Check sheet for the modelled part. Datum: model origin and axes. Units: mm. Face numbers are marked on the shaded views. Give positions to 0.01 mm unless a question says otherwise; leave off trailing zeros. Order: outer loops, then holes, each group sorted by start corner. A loop starts at its lowest first (then second) coordinate and runs counter-clockwise, first axis right, second up.
```python
from build123d import *

# Parameters (mm, degrees)
SKETCH1_R           = 10.308435719
BOSS_EXTRUDE1_DEPTH = 6


with BuildPart() as part:
    # Sketch1 → Boss-Extrude1 (new body)
    with BuildSketch(Plane(origin=(0, 0, 0), x_dir=(1, 0, 0), z_dir=(0, 1, 0))):
        Polygon((9.406647228, 13.324720403), (37.205859161, 61.474367881), (61.474367881, 37.205859161), (13.324720403, 9.406647228), (14.808755665, 6.836222753), (62.958403143, 34.635434686), (71.841293847, 1.484035262), (16.242869981, 1.484035262), (16.242869981, -1.484035262), (71.841293847, -1.484035262), (62.958403143, -34.635434686), (14.808755665, -6.836222753), (13.324720403, -9.406647228), (61.474367881, -37.205859161), (37.205859161, -61.474367881), (9.406647228, -13.324720403), (6.836222753, -14.808755665), (34.635434686, -62.958403143), (1.484035262, -71.841293847), (1.484035262, -16.242869981), (-1.484035262, -16.242869981), (-1.484035262, -71.841293847), (-34.635434686, -62.958403143), (-6.836222753, -14.808755665), (-9.406647228, -13.324720403), (-37.205859161, -61.474367881), (-61.474367881, -37.205859161), (-13.324720403, -9.406647228), (-14.808755665, -6.836222753), (-62.958403143, -34.635434686), (-71.841293847, -1.484035262), (-16.242869981, -1.484035262), (-16.242869981, 1.484035262), (-71.841293847, 1.484035262), (-62.958403143, 34.635434686), (-14.808755665, 6.836222753), (-13.324720403, 9.406647228), (-61.474367881, 37.205859161), (-37.205859161, 61.474367881), (-9.406647228, 13.324720403), (-6.836222753, 14.808755665), (-34.635434686, 62.958403143), (-1.484035262, 71.841293847), (-1.484035262, 16.242869981), (1.484035262, 16.242869981), (1.484035262, 71.841293847), (34.635434686, 62.958403143), (6.836222753, 14.808755665), align=None)
        with Locations(Location((0, 0, 0), (0, 0, 270))):
            Circle(SKETCH1_R, mode=Mode.SUBTRACT)
    extrude(amount=-BOSS_EXTRUDE1_DEPTH)


solid = part.part
```
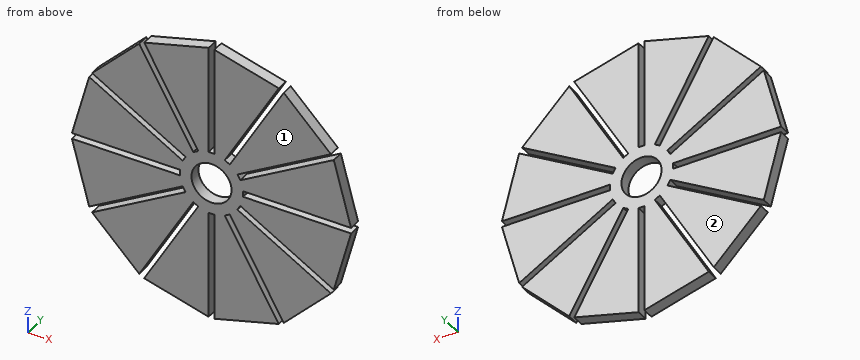
(1) Gauge pin test, flat ends, axial feed: pin 1 Ø3.5 at (y, z) = (-2, 0) entering from +X; pin 2 Ø0.9 at (x, y) = (0.5, -3) entering from -Z; pin 3 Ø18.5 at (x, z) = (0, 0) entering from +Y; pin 4 Ø3 at (y, z) = (-2.5, 22.5) entering from -X. Record the tip position at first contact, or that the pin passes through.
Response values:
pin 1: stops at x = 71.84
pin 2: stops at z = -16.24
pin 3: passes through
pin 4: stops at x = -66.61
(2) Cross-section at B-B on x = -23. Enter the section's corners in (y, z), then the cut area to 3 significant figures.
Response values:
outline: (-6, -66.08) - (0, -66.08) - (0, -42.81) - (-6, -42.81) - close; (-6, -36.87) - (0, -36.87) - (0, -14.99) - (-6, -14.99) - close; (-6, -11.57) - (0, -11.57) - (0, -1.48) - (-6, -1.48) - close; (-6, 1.48) - (0, 1.48) - (0, 11.57) - (-6, 11.57) - close; (-6, 14.99) - (0, 14.99) - (0, 36.87) - (-6, 36.87) - close; (-6, 42.81) - (0, 42.81) - (0, 66.08) - (-6, 66.08) - close
area: 663 mm2
(3) Release check for a two-part mould opening along Y. For the marked faces 1 and 2 record: released by +Y, released by -Y, zero draft, split by the parting line, or undercut.
Response values:
face 1: released by -Y
face 2: released by +Y
(4) Material ranges on L1, parallel to X at y = -4.35, z = 0; L2, parallel to Z at x = -55.5, y = -3.35; L3, parallel to Z at x = 14.5, y = -0.95, recorded low to high.
Response values:
L1: x = -16.24 to -10.31, 10.31 to 16.24
L2: z = -43.18 to -33.76, -30.33 to -1.48, 1.48 to 30.33, 33.76 to 43.18
L3: z = -68.35 to -28.08, -22.15 to -10.09, -7.37 to 7.37, 10.09 to 22.15, 28.08 to 68.35
(5) Cross-section at A-A on z = 32. Enter the section's corners in (x, y).
Response values:
outline: (-63.66, -6) - (-58.39, -6) - (-58.39, 0) - (-63.66, 0) - close; (-52.46, -6) - (-20.19, -6) - (-20.19, 0) - (-52.46, 0) - close; (-16.76, -6) - (-1.48, -6) - (-1.48, 0) - (-16.76, 0) - close; (1.48, -6) - (16.76, -6) - (16.76, 0) - (1.48, 0) - close; (20.19, -6) - (52.46, -6) - (52.46, 0) - (20.19, 0) - close; (58.39, -6) - (63.66, -6) - (63.66, 0) - (58.39, 0) - close
